Work out the finished part from the listing and answer in its coordinate system (mm). Give positions to 0.01 mm unless a question says otherwise; leave off trailing zeros. Order: outer loops, then holes, each group sorted by start corner. A loop starts at its lowest first (then second) coordinate and runs counter-clockwise, first axis right, second up. Notation, with made-up numbers: (-8.75, 89.25) - (46.25, 89.25) arc R17 ccw to (46.25, 101.25) - close; hole circle Ø9 at (-27.75, -36.5). An arc over 180 degrees is marked (long way). Return JSON: item names as keys, results as strings. Group by question number.
from build123d import *

# Parameters (mm, degrees)
SKETCH1_W           = 38
SKETCH1_H           = 44
SKETCH1_R           = 2
BOSS_EXTRUDE1_DEPTH = 2.5


with BuildPart() as part:
    # Sketch1 → Boss-Extrude1 (new, symmetric)
    with BuildSketch(Plane.XY):
        Rectangle(SKETCH1_W, SKETCH1_H)
        with Locations((-15, 16)):
            Circle(SKETCH1_R, mode=Mode.SUBTRACT)
        with Locations(Location((-15, -16, 0), (0, 0, 180))):
            Circle(SKETCH1_R, mode=Mode.SUBTRACT)
        with Locations((15, -16)):
            Circle(SKETCH1_R, mode=Mode.SUBTRACT)
        with Locations(Location((15, 16, 0), (0, 0, 180))):
            Circle(SKETCH1_R, mode=Mode.SUBTRACT)
    extrude(amount=BOSS_EXTRUDE1_DEPTH, both=True)


solid = part.part
1. The part is cut by section A-A (x = -15). Give the vertices of the cut face in (y, z), and give its area (3 significant figures).
2. The part is cut by section C-C (z = -1.85). Give the vertices of the cut face in (x, y).
3. The part is cut by section B-B (y = 16). Give the vertices of the cut face in (x, z), and give its area (3 significant figures).
4. Consider probe 1 along Y at (x, z) = (15, -1.15); probe 2 along X at (y, z) = (-15, -1.6); probe 3 along X at (y, z) = (16.5, 1). Determine where each line is inside the solid, lowest interval first. Write a range as from..to.
5. Determine the mould class of faces 1 (the cylindrical face through (-15, -18, 0)), 2 (the cylindrical face through (-15, 18, 0)), 3 (the flat face through (19, 0, 0)), 4 (the flat face through (0, -22, 0)) for opening direction Y: released by +Y, released by -Y, zero draft, split by the parting line, or undercut.
Answers:
{
 "1": {"outline": "(-22, -2.5) - (-18, -2.5) - (-18, 2.5) - (-22, 2.5) - close; (-14, -2.5) - (14, -2.5) - (14, 2.5) - (-14, 2.5) - close; (18, -2.5) - (22, -2.5) - (22, 2.5) - (18, 2.5) - close", "area": "180 mm^2"},
 "2": {"outline": "(-19, -22) - (19, -22) - (19, 22) - (-19, 22) - close; hole circle Ø4 at (-15, -16); hole circle Ø4 at (-15, 16); hole circle Ø4 at (15, -16); hole circle Ø4 at (15, 16)"},
 "3": {"outline": "(-19, -2.5) - (-17, -2.5) - (-17, 2.5) - (-19, 2.5) - close; (-13, -2.5) - (13, -2.5) - (13, 2.5) - (-13, 2.5) - close; (17, -2.5) - (19, -2.5) - (19, 2.5) - (17, 2.5) - close", "area": "150 mm^2"},
 "4": {"probe 1": "y = -22..-18, -14..14, 18..22", "probe 2": "x = -19..-16.73, -13.27..13.27, 16.73..19", "probe 3": "x = -19..-16.94, -13.06..13.06, 16.94..19"},
 "5": {"face 1": "undercut", "face 2": "undercut", "face 3": "zero draft", "face 4": "released by -Y"}
}
